Build history of the part. All positions in model axes, mm. Face numbers are marked on the shaded views. A direction names the side the tool comes from. Coordinates: 2 decimals unless noted, no trailing zeros. Return JSON: item names as keys, results as strings.
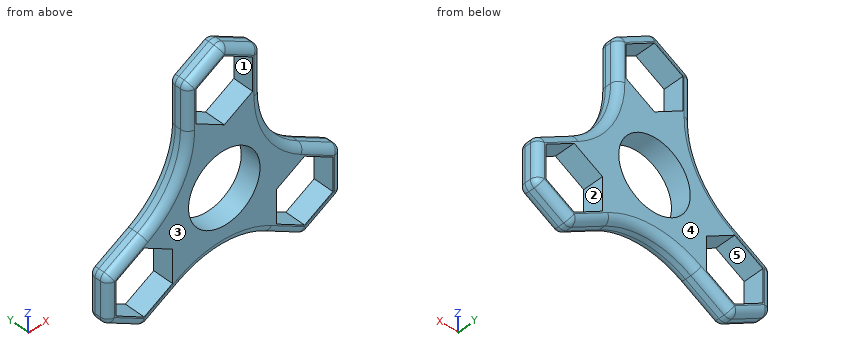
from build123d import *

# Parameters (mm, degrees)
F0_R     = 14.2875
F0_R_2   = 11.0236
F1_DEPTH = 6.35
F2_R     = 2.286


with BuildPart() as f1:
    # F0 (on Front) → F1 (new body)
    with BuildSketch(Plane.XZ):
        Polygon((-11.43, 35.174114), (-11.43, 21.975886), (0, 15.376773), (11.43, 21.975886), (11.43, 35.174114), (0, 41.773227), align=None)
        Polygon((0, 18.485689), (-8.7376, 23.530344), (-8.7376, 33.619656), (0, 38.664311), (8.7376, 33.619656), (8.7376, 23.530344), align=None, mode=Mode.SUBTRACT)
        with BuildLine():
            Line((0, 15.376773), (-11.43, 21.975886))
            ThreePointArc((-11.43, 21.975886), (-14.966436, 8.660036), (-24.701385, -1.089272))
            Line((-24.701385, -1.089272), (-13.271385, -7.688386))
            Line((-13.271385, -7.688386), (-13.271385, -20.886613))
            ThreePointArc((-13.271385, -20.886613), (0.028698, -17.291331), (13.339321, -20.84739))
            Line((13.339321, -20.84739), (13.339321, -7.649163))
            Line((13.339321, -7.649163), (24.769321, -1.050049))
            ThreePointArc((24.769321, -1.050049), (15.023862, 8.681056), (11.43, 21.975886))
            Line((11.43, 21.975886), (0, 15.376773))
        make_face()
        Circle(F0_R, mode=Mode.SUBTRACT)
        Polygon((-13.271385, -7.688386), (-24.701385, -1.089272), (-36.131385, -7.688386), (-36.131385, -20.886613), (-24.701385, -27.485727), (-13.271385, -20.886613), align=None)
        Polygon((-24.701385, -24.376811), (-33.438985, -19.332155), (-33.438985, -9.242844), (-24.701385, -4.198188), (-15.963785, -9.242844), (-15.963785, -19.332155), align=None, mode=Mode.SUBTRACT)
        Polygon((36.199321, -7.649163), (24.769321, -1.050049), (13.339321, -7.649163), (13.339321, -20.84739), (24.769321, -27.446504), (36.199321, -20.84739), align=None)
        Polygon((33.506921, -9.203621), (33.506921, -19.292932), (24.769321, -24.337588), (16.031721, -19.292932), (16.031721, -9.203621), (24.769321, -4.158965), align=None, mode=Mode.SUBTRACT)
        Circle(F0_R)
        Circle(F0_R_2, mode=Mode.SUBTRACT)
    extrude(amount=F1_DEPTH)

    # F2
    f2_edges = [f1.edges().sort_by_distance(p)[0] for p in [
        (0.028698, -6.35, -17.291331),
        (30.484321, -6.35, -24.146947),
        (36.199321, -6.35, -14.248276),
        (15.023862, -6.35, 8.681056),
        (11.43, -6.35, 28.575),
        (5.715, -6.35, 38.47367),
        (-5.715, -6.35, 38.47367),
        (-11.43, -6.35, 28.575),
        (-14.966436, -6.35, 8.660036),
        (-36.131385, -6.35, -14.2875),
        (-30.416385, -6.35, -24.18617),
        (-18.986385, -6.35, -24.18617),
        (-36.131385, 0, -14.2875),
        (-30.416385, 0, -4.388829),
        (-11.43, 0, 28.575),
        (-5.715, 0, 38.47367),
        (5.715, 0, 38.47367),
        (30.484321, -6.35, -4.349606),
        (11.43, 0, 28.575),
        (15.023862, 0, 8.681056),
        (0.028698, 0, -17.291331),
        (30.484321, 0, -24.146947),
        (19.054321, 0, -24.146947),
        (-30.416385, -6.35, -4.388829),
        (19.054321, -6.35, -24.146947),
        (-30.416385, 0, -24.18617),
        (36.199321, 0, -14.248276),
        (-14.966436, 0, 8.660036),
        (30.484321, 0, -4.349606),
        (-18.986385, 0, -24.18617),
        (0, -3.175, 41.773227),
        (-11.43, -3.175, 35.174114),
        (-11.43, -3.175, 21.975886),
        (-36.131385, -3.175, -7.688386),
        (-36.131385, -3.175, -20.886613),
        (-24.701385, -3.175, -27.485727),
        (24.769321, -3.175, -27.446504),
        (36.199321, -3.175, -20.84739),
        (36.199321, -3.175, -7.649163),
        (11.43, -3.175, 35.174114),
    ]]
    fillet(f2_edges, radius=F2_R)


solid = f1.part
1. Cut at A-A on y = -5. State how many separate pieces and enclosed holes the cut face has, plus the area to 3 significant figures.
Check values:
{"separate pieces": "1", "enclosed holes": "4", "area": "1,300 mm²"}
2. Drop flat-ended pins along their axis: pin 1 (20 mm diameter, centred on x = 0, z = 0, fed in from +Y); pin 2 (0.5 mm diameter, centred on y = -3, z = 26, fed in from -X); pin 3 (3 mm diameter, centred on y = -5.5, z = -4, fed in from -X); pin 4 (1.5 mm diameter, centred on x = 10.5, y = -4, fed in from -Z). Give the stop position or say it passes through.
Check values:
{"pin 1": "through", "pin 2": "x = -11.43", "pin 3": "x = -31.81", "pin 4": "z = -19.76"}
3. Probe L1, parallel to Z at x = 0, y = -4; L2, parallel to X at y = -5, z = -5; L3, parallel to X at y = -1.5, z = -5. List the from-to ranges inside material, lowest first.
Check values:
{"L1": "-17.29 to -11.02, 11.02 to 18.49, 38.66 to 41.42", "L2": "-31.07 to -26.09, -23.31 to -9.82, 9.82 to 23.31, 26.23 to 31.21", "L3": "-31.2 to -26.09, -23.31 to -9.82, 9.82 to 23.31, 26.23 to 31.33"}
4. Mould opens along X. For the marked faces 1, 2 and 3 say: pulls with the +X half, pulls with the -X half, needs draft (parallel to the pull), parting line crosses it, or undercut.
Check values:
{"face 1": "undercut", "face 2": "undercut", "face 3": "needs draft"}
5. Tool access for the marked faces 4 and 5: list every direction of +Z, -Z, +X, -X, +Y, -Y with a clear straight run to the whole face (end or side of a thin tool).
Check values:
{"face 4": "+Z, -Z, +X, -X, +Y", "face 5": "+Y, -Y"}
